Geometry: final body of the model. Coordinates: model frame, mm. A direction names the side the tool comes from. Give positions to 0.01 mm unless a question says otherwise; leave off trailing zeros. Write each loop counter-clockwise with the first axis right and the second up, starting at its lowest first coordinate (ties: lowest second). Pieces come first, ordered by that corner, then holes. Notation, with made-up numbers: M 70.25,68.25 L 128.25,68.25 A22 ccw 128.25,92.25 Z; hole C 50,-5 d8. An arc over 180 degrees is marked long. Use a Markdown table: item, result. Add a question column.
(1) Reachability of faces 4 (the cylindrical face through (2.46, 3.96, 4.14)), 5 (the cylindrical face through (0.402, 0.507, 9.986)), 6 (the flat face through (4, 13, 13)) from +Z, -Z, +X, -X, +Y, -Y: full face, straight path, thin tool, end or side. Return the list, or none.
(2) Cut plane B-B (x = 4). Output: boundary loops of the cut face in (y, z).
(3) Cut plane C-C (z = 2). Output: boundary loops of the cut face in (x, y).
(4) Cut plane A-A (y = 3.5). Output: boundary loops of the cut face in (x, z).
(5) Material intervals for L1, parallel to X at y = 11.75, z = 7.75; L2, parallel to Z at x = 10, y = 7.25; L3, parallel to Z at x = 1.5, y = 5.25, sorted ascending.
(6) Draft query along X for faces 1 (the flat face through (5, 0, 7)), 2 (the flat face through (7.5, 0.5, 5.845)), 3 (the flat face through (-1.5, 6, 7)). Return one class per face: released by +X, released by -X, zero draft, split by the parting line, or undercut.
(7) Pin query (flat end, axial travel): pin 1 Ø2 at (x, z) = (9, 6) entering from +Y; pin 2 Ø2.5 at (x, z) = (3, 6.5) entering from +Y. Return the tip coordinate at first contact, or that it passes through.
```python
from build123d import *

# Parameters (mm, degrees)
SKETCH1_W           = 13
SKETCH1_H           = 13
SKETCH1_W_2         = 12
SKETCH1_H_2         = 12
BOSS_EXTRUDE1_DEPTH = 13
SKETCH1_4_W         = 12
SKETCH1_4_H         = 12
SKETCH1_4_W_2       = 6
SKETCH1_4_H_2       = 8
SKETCH1_4_W_3       = 4
SKETCH1_4_H_3       = 1.754040625
BOSS_EXTRUDE2_DEPTH = 1
SKETCH1_7_W         = 6
SKETCH1_7_H         = 8
SKETCH1_7_W_2       = 4
SKETCH1_7_H_2       = 1.754040625
CUT_EXTRUDE1_DEPTH  = 1
FILLET1_R           = 3
SKETCH3_W           = 0.743374663
SKETCH3_H           = 1.154040625
SKETCH3_W_2         = 0.3
BOSS_EXTRUDE3_DEPTH = 1
FILLET2_R           = 20
BOSS_EXTRUDE4_DEPTH = 6


# Some blends are built 0.0001 mm under size
with BuildPart() as part:
    # Sketch1 → Boss-Extrude1 (new body)
    with BuildSketch(Plane(origin=(0, 0, 0), x_dir=(1, 0, 0), z_dir=(0, 1, 0))):
        with Locations((5, -6.841440964)):
            Rectangle(SKETCH1_W, SKETCH1_H)
        with Locations((5, -6.841440964)):
            Rectangle(SKETCH1_W_2, SKETCH1_H_2, mode=Mode.SUBTRACT)
    extrude(amount=BOSS_EXTRUDE1_DEPTH)

    # Sketch1<4> → Boss-Extrude2 (add)
    # profile 1 of 3: a face of its own
    with BuildSketch(Plane(origin=(0, 0, 0), x_dir=(1, 0, 0), z_dir=(0, 1, 0))):
        with Locations((5, -6.841440964)):
            Rectangle(SKETCH1_4_W, SKETCH1_4_H)
        Polygon((-0.500000048, -10.841440964), (-0.500000048, -2.841440964), (5.499999952, -2.841440964), (5.499999952, -5.84487475), (9.499999952, -5.84487475), (9.499999952, -7.598915375), (5.499999952, -7.598915375), (5.499999952, -10.841440964), align=None, mode=Mode.SUBTRACT)
    # profile 2 of 3: a face of its own
    with BuildSketch(Plane(origin=(0, 0, 0), x_dir=(1, 0, 0), z_dir=(0, 1, 0))):
        with Locations((2.499999952, -6.841440964)):
            Rectangle(SKETCH1_4_W_2, SKETCH1_4_H_2)
    # profile 3 of 3: a face of its own
    with BuildSketch(Plane(origin=(0, 0, 0), x_dir=(1, 0, 0), z_dir=(0, 1, 0))):
        with Locations((7.499999952, -6.721895063)):
            Rectangle(SKETCH1_4_W_3, SKETCH1_4_H_3)
    extrude(amount=BOSS_EXTRUDE2_DEPTH)

    # Sketch1<7> → Cut-Extrude1 (cut)
    with BuildSketch(Plane(origin=(0, 0, 0), x_dir=(1, 0, 0), z_dir=(0, 1, 0))):
        with Locations((2.499999952, -6.841440964)):
            Rectangle(SKETCH1_7_W, SKETCH1_7_H)
        with Locations((7.499999952, -6.721895063)):
            Rectangle(SKETCH1_7_W_2, SKETCH1_7_H_2)
    extrude(amount=CUT_EXTRUDE1_DEPTH, mode=Mode.SUBTRACT)

    # Fillet1
    fillet1_edges = [part.edges().sort_by_distance(p)[0] for p in [
        (5.499999952, 0.5, 2.841440964),
        (-0.500000048, 0.5, 2.841440964),
        (-0.500000048, 0.5, 10.841440964),
        (5.499999952, 0.5, 10.841440964),
    ]]
    fillet(fillet1_edges, radius=FILLET1_R - 0.0001)  # a hair under: the kernel refuses the full size

    # Sketch3 → Boss-Extrude3 (add)
    with BuildSketch(Plane.XZ):
        with Locations((9.871687284, 6.721895063)):
            Rectangle(SKETCH3_W, SKETCH3_H)
        with BuildLine():
            Line((5.199999952, 7.298915375), (5.199999952, 7.841440964))
            ThreePointArc((5.199999952, 7.841440964), (4.409188261, 9.750629273), (2.499999952, 10.541440964))
            ThreePointArc((2.499999952, 10.541440964), (0.590811643, 9.750629273), (-0.200000048, 7.841440964))
            Line((-0.200000048, 7.841440964), (-0.200000048, 5.841440964))
            ThreePointArc((-0.200000048, 5.841440964), (0.590811643, 3.932252654), (2.499999952, 3.141440964))
            ThreePointArc((2.499999952, 3.141440964), (4.409188261, 3.932252654), (5.199999952, 5.841440964))
            Line((5.199999952, 5.841440964), (5.199999952, 6.14487475))
            Line((5.199999952, 6.14487475), (9.199999952, 6.14487475))
            Line((9.199999952, 6.14487475), (9.199999952, 7.298915375))
            Line((9.199999952, 7.298915375), (5.199999952, 7.298915375))
        make_face()
        with Locations((9.349999952, 6.721895063)):
            Rectangle(SKETCH3_W_2, SKETCH3_H)
    extrude(amount=-BOSS_EXTRUDE3_DEPTH)

    # Fillet2
    # the kernel refuses this fillet: 20 mm, written as the material it adds along each edge
    with BuildSketch(Plane(origin=(9.499999952, 0, 7.298915375), x_dir=(0, 0, 1), z_dir=(0, 1, 0)), Plane(origin=(9.499999952, 1, 6.14487475), x_dir=(0, 0, -1), z_dir=(0, -1, 0))) as fillet2_piece_1:
        with BuildLine():
            CenterArc((20, -3.451086785), FILLET2_R, 170.063632928, 9.936367072)
            Line((0, -3.451086785), (0, 0))
            Line((0, 0), (0.3, 0))
        make_face()
    extrude(amount=1)

    # Sketch4 → Boss-Extrude4 (add)
    with BuildSketch(Plane(origin=(0, 1, 0), x_dir=(1, 0, 0), z_dir=(0, 1, 0))):
        with BuildLine():
            Line((4.199999952, -5.841440964), (4.199999952, -7.841440964))
            ThreePointArc((4.199999952, -7.841440964), (2.499999952, -9.541440964), (0.799999952, -7.841440964))
            Line((0.799999952, -7.841440964), (0.799999952, -5.841440964))
            ThreePointArc((0.799999952, -5.841440964), (2.499999952, -4.141440964), (4.199999952, -5.841440964))
        make_face()
    extrude(amount=BOSS_EXTRUDE4_DEPTH)


solid = part.part
```
Answer list:
| question | item | result |
|---|---|---|
| 1 | face 4 | +Y |
| 1 | face 5 | +Y, -Y |
| 1 | face 6 | +Z, -Z, +X, -X, +Y |
| 2 | outline | M 0,0.34 L 13,0.34 L 13,0.84 L 1,0.84 L 1,3.24 L 0,3.24 Z; M 0,3.6 L 1,3.6 L 1,5.04 L 7,5.04 L 7,8.64 L 1,8.64 L 1,10.09 L 0,10.09 Z; M 0,10.44 L 1,10.44 L 1,12.84 L 13,12.84 L 13,13.34 L 0,13.34 Z |
| 3 | outline | M -1.5,0 L 11.5,0 L 11.5,13 L 11,13 L 11,1 L -1,1 L -1,13 L -1.5,13 Z |
| 4 | outline | M -1.5,0.34 L 11.5,0.34 L 11.5,13.34 L -1.5,13.34 Z; M 0.8,5.84 A1.7 ccw 4.2,5.84 L 4.2,7.84 A1.7 ccw 0.8,7.84 Z; hole M -1,0.84 L 11,0.84 L 11,12.84 L -1,12.84 Z |
| 5 | L1 | -1.5 to -1, 11 to 11.5 |
| 5 | L2 | 0.34 to 0.84, 12.84 to 13.34 |
| 5 | L3 | 0.34 to 0.84, 4.47 to 9.22, 12.84 to 13.34 |
| 6 | face 1 | zero draft |
| 6 | face 2 | undercut |
| 6 | face 3 | released by -X |
| 7 | pin 1 | y = 1 |
| 7 | pin 2 | y = 7 |
